Check sheet for the modelled part. Datum: model origin and axes. Units: mm. Face numbers are marked on the shaded views. A direction names the side the tool comes from. Give positions to 0.01 mm unless a question says otherwise; leave off trailing zeros. Order: outer loops, then holes, each group sorted by start corner. A loop starts at its lowest first (then second) coordinate and runs counter-clockwise, first axis right, second up.
```python
from build123d import *

# Parameters (mm, degrees)
SKETCH1_W           = 16
SKETCH1_H           = 40
BOSS_EXTRUDE1_DEPTH = 2
FILLET1_R           = 5
FILLET2_R           = 2
BOSS_EXTRUDE2_DEPTH = 25


with BuildPart() as part:
    # Sketch1 → Boss-Extrude1 (new body)
    with BuildSketch(Plane(origin=(0, 0, 0), x_dir=(1, 0, 0), z_dir=(0, 1, 0))):
        Polygon((32.5, -19), (38.5, -25), (62.5, -25), (62.5, 25), (38.5, 25), (32.5, 19), (-32.5, 19), (-32.5, -19), align=None)
        with Locations((48, 0)):
            Rectangle(SKETCH1_W, SKETCH1_H, mode=Mode.SUBTRACT)
    extrude(amount=BOSS_EXTRUDE1_DEPTH)

    # Fillet1
    fillet1_edges = [part.edges().sort_by_distance(p)[0] for p in [
        (32.5, 1, -19),
        (38.5, 1, -25),
        (62.5, 1, -25),
        (62.5, 1, 25),
        (38.5, 1, 25),
        (32.5, 1, 19),
    ]]
    fillet(fillet1_edges, radius=FILLET1_R)

    # Fillet2
    fillet2_edges = [part.edges().sort_by_distance(p)[0] for p in [
        (40, 1, -20),
        (40, 1, 20),
        (56, 1, 20),
        (56, 1, -20),
    ]]
    fillet(fillet2_edges, radius=FILLET2_R)

    # Sketch2 → Boss-Extrude2 (add, symmetric)
    with BuildSketch(Plane.XY):
        with BuildLine():
            Line((46, 0), (50, 0))
            Line((50, 0), (51, 1))
            Line((51, 1), (51, 2))
            ThreePointArc((51, 2), (48, 3.605551275), (45, 2))
            Line((45, 2), (45, 1))
            Line((45, 1), (46, 0))
        make_face()
    extrude(amount=BOSS_EXTRUDE2_DEPTH, both=True)


solid = part.part
```
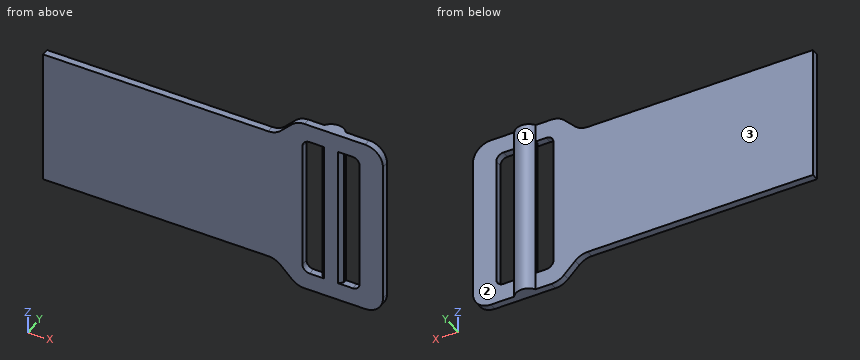
(1) Cross-section at A-A on x = 52.5. Enter the section's corners in (y, z), then the cut area to 3 significant figures.
Response values:
outline: (0, -25) - (2, -25) - (2, -20) - (0, -20) - close; (0, 20) - (2, 20) - (2, 25) - (0, 25) - close
area: 20.0 mm2
(2) Cross-section at C-C on x = 26.5. Enter the section's corners in (y, z), then the cut area to 3 significant figures.
Response values:
outline: (0, -19) - (2, -19) - (2, 19) - (0, 19) - close
area: 76.0 mm2
(3) Cross-section at D-D on y = 2.7. Enter the section's corners in (x, z).
Response values:
outline: (45.61, -25) - (50.39, -25) - (50.39, 25) - (45.61, 25) - close
(4) Gauge pin test, flat ends, axial feed: pin 1 Ø1 at (x, z) = (19, -17) entering from +Y; pin 2 Ø0.6 at (x, y) = (-13, 1) entering from -Z; pin 3 Ø1.6 at (x, y) = (14, 1) entering from +Z. Record the tip position at first contact, or that the pin passes through.
Response values:
pin 1: stops at y = 2
pin 2: stops at z = -19
pin 3: stops at z = 19
(5) Set-up check for the marked faces 1, 2 and 3: record each of +Z, -Z, +X, -X, +Y, -Y from which the full face is reachable in a straight line by a thin tool's end or side.
Response values:
face 1: +Z, -Z, +Y
face 2: +Z, -Z, +X, +Y
face 3: +Z, -Z, -X, +Y
(6) Cross-section at B-B on z = -5.5. Enter the section's corners in (x, y), then the cut area to 3 significant figures.
Response values:
outline: (-32.5, 0) - (40, 0) - (40, 2) - (-32.5, 2) - close; (45, 1) - (46, 0) - (50, 0) - (51, 1) - (51, 2) arc R3.61 ccw to (45, 2) - close; (56, 0) - (62.5, 0) - (62.5, 2) - (56, 2) - close
area: 176 mm2
(7) Material ranges on L1, parallel to X at y = 1.3, z = 15.5; L2, parallel to X at y = 0.45, z = 14.5; L3, parallel to Z at x = -13.5, y = 0.55, recorded low to high.
Response values:
L1: x = -32.5 to 40, 45 to 51, 56 to 62.5
L2: x = -32.5 to 40, 45.55 to 50.45, 56 to 62.5
L3: z = -19 to 19
